CAD build for the part. Positions are in the model's coordinates, mm. Give positions to 0.01 mm unless a question says otherwise; leave off trailing zeros. Order: outer loops, then holes, each group sorted by start corner. A loop starts at its lowest first (then second) coordinate and runs counter-clockwise, first axis right, second up. Notation, with made-up numbers: (20.25, 22.5) -> (28.25, 22.5) arc R22 ccw to (28.25, 30.5) -> close; hole circle Ø10 at (34, 72). An arc over 180 degrees is marked (long way). Use one line per item in the form item = value. Start each with the question number.
1) Probe line 1 (X direction, y = 0, z = -26); line 2 (Y direction, x = -55, z = 31.5); line 3 (X direction, y = 4.75, z = -13.5). List the from-to ranges inside material, lowest first.
2) Cut at B-B, the plane z = 26.5. Give the cut face in (x, y), and give its area (3 significant figures).
3) Drop flat-ended pins along their axis: P1, Ø8, axis at x = 200, y = 0, coming from the +Z side; P2, Ø5, axis at x = -55, y = 0, coming from the +Z side; P3, Ø5, axis at y = 5.5, z = 16.5, coming from the +X side. Give the stop position or say it passes through.
4) Cut at A-A, the plane x = 235. Give the cut face in (y, z).
from build123d import *

# Parameters (mm, degrees)
F1_DEPTH = 9
F2_R     = 5.5
F3_DEPTH = 51
F4_R     = 2.1
F5_DEPTH = 25
F6_R     = 5
F7_DEPTH = 25
F8_SIZE  = 5
F9_SIZE  = 2.1
F10_SIZE = 0.5


with BuildPart() as f1:
    # F0 (on Front) → F1 (new body, symmetric)
    with BuildSketch(Plane.XZ):
        Polygon((-245, 13.5), (-245, -37.5), (245, -37.5), (245, 13.5), (150, 13.5), (150, 37.5), (-150, 37.5), (-150, 13.5), align=None)
    extrude(amount=F1_DEPTH, both=True)

    # F2 (on face) → F3 (cut, through all)
    with BuildSketch(Plane(origin=(0, 0, -37.5), x_dir=(1, 0, 0), z_dir=(0, 0, -1))):
        with Locations((235, 0)):
            Circle(F2_R)
        with Locations((165, 0)):
            Circle(F2_R)
        with Locations((-165, 0)):
            Circle(F2_R)
        with Locations((-235, 0)):
            Circle(F2_R)
    extrude(amount=-F3_DEPTH, mode=Mode.SUBTRACT)

    # F4 (on face) → F5 (cut)
    with BuildSketch(Plane.XY.offset(37.5)):
        with Locations((-115, 0)):
            Circle(F4_R)
        with Locations((-55, 0)):
            Circle(F4_R)
        with Locations((5, 0)):
            Circle(F4_R)
        with Locations((65, 0)):
            Circle(F4_R)
        with Locations((125, 0)):
            Circle(F4_R)
    extrude(amount=-F5_DEPTH, mode=Mode.SUBTRACT)

    # F6 (on face) → F7 (cut)
    with BuildSketch(Plane.XY.offset(13.5)):
        with Locations((-200, 0)):
            Circle(F6_R)
        with Locations((200, 0)):
            Circle(F6_R)
    extrude(amount=-F7_DEPTH, mode=Mode.SUBTRACT)

    # F8
    f8_edges = [f1.edges().sort_by_distance(p)[0] for p in [
        (-205, 0, -11.5),
        (195, 0, -11.5),
    ]]
    chamfer(f8_edges, length=F8_SIZE)

    # F9
    f9_edges = [f1.edges().sort_by_distance(p)[0] for p in [
        (122.9, 0, 12.5),
        (62.9, 0, 12.5),
        (2.9, 0, 12.5),
        (-57.1, 0, 12.5),
        (-117.1, 0, 12.5),
    ]]
    chamfer(f9_edges, length=F9_SIZE)

    # F10
    f10_edges = [f1.edges().sort_by_distance(p)[0] for p in [
        (-159.5, 0, -12),
        (-170.5, 0, -37.5),
        (-170.5, 0, 13.5),
        (-229.5, 0, -12),
        (-240.5, 0, -37.5),
        (-240.5, 0, 13.5),
        (-205, 0, 13.5),
        (-117.1, 0, 37.5),
        (-57.1, 0, 37.5),
        (2.9, 0, 37.5),
        (62.9, 0, 37.5),
        (122.9, 0, 37.5),
        (170.5, 0, -12),
        (159.5, 0, -37.5),
        (159.5, 0, 13.5),
        (240.5, 0, -12),
        (229.5, 0, -37.5),
        (229.5, 0, 13.5),
        (195, 0, 13.5),
    ]]
    chamfer(f10_edges, length=F10_SIZE)


solid = f1.part
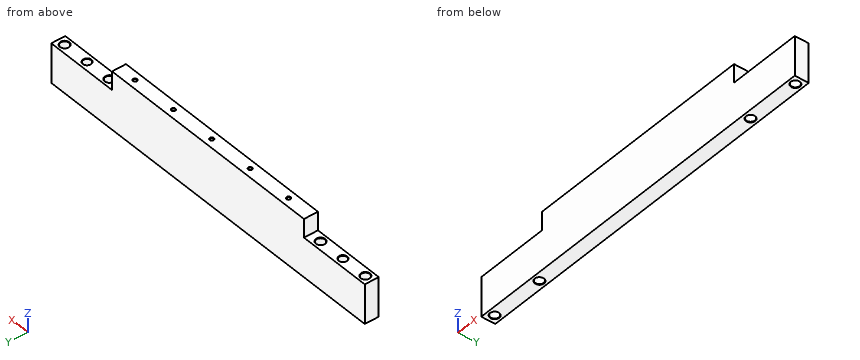
Result:
q1.line_1 = -245 to -240.5, -229.5 to -170.5, -159.5 to 159.5, 170.5 to 229.5, 240.5 to 245
q1.line_2 = -9 to -2.1, 2.1 to 9
q1.line_3 = -245 to -237.77, -232.23 to -167.77, -162.23 to 162.23, 167.77 to 232.23, 237.77 to 245
q2.outline = (-150, -9) -> (150, -9) -> (150, 9) -> (-150, 9) -> close; hole circle Ø4.2 at (-115, 0); hole circle Ø4.2 at (-55, 0); hole circle Ø4.2 at (5, 0); hole circle Ø4.2 at (65, 0); hole circle Ø4.2 at (125, 0)
q2.area = 5,330 mm²
q3.P1 = -7.5
q3.P2 = 37.4
q3.P3 = 150
q4.outline = (-9, -37.5) -> (-6, -37.5) -> (-5.5, -37) -> (-5.5, 13) -> (-6, 13.5) -> (-9, 13.5) -> close; (5.5, -37) -> (6, -37.5) -> (9, -37.5) -> (9, 13.5) -> (6, 13.5) -> (5.5, 13) -> close
